from build123d import *

# Parameters (mm, degrees)
SKETCH1_R           = 1.5
SKETCH1_W           = 30
SKETCH1_H           = 8
BOSS_EXTRUDE1_DEPTH = 1.6
SKETCH1_3_W         = 30
SKETCH1_3_H         = 8
BOSS_EXTRUDE2_DEPTH = 11.9


with BuildPart() as part:
    # Sketch1 → Boss-Extrude1 (new body)
    # profile 1 of 2: a face of its own
    with BuildSketch(Plane(origin=(0, 0, 0), x_dir=(0, 1, 0), z_dir=(0, 0, 1))):
        with BuildLine():
            ThreePointArc((0, 2.5), (0.732233047, 0.732233047), (2.5, 0))
            Line((2.5, 0), (5.875, 0))
            Line((5.875, 0), (5.875, 8))
            Line((5.875, 8), (35.875, 8))
            Line((35.875, 8), (35.875, 0))
            Line((35.875, 0), (39.25, 0))
            ThreePointArc((39.25, 0), (41.017766953, 0.732233047), (41.75, 2.5))
            Line((41.75, 2.5), (41.75, 45.6))
            ThreePointArc((41.75, 45.6), (41.017766953, 47.367766953), (39.25, 48.1))
            Line((39.25, 48.1), (2.5, 48.1))
            ThreePointArc((2.5, 48.1), (0.732233047, 47.367766953), (0, 45.6))
            Line((0, 45.6), (0, 2.5))
        make_face()
        with Locations(Location((2.549913685, 2.549913685, 0), (0, 0, 270))):
            Circle(SKETCH1_R, mode=Mode.SUBTRACT)
        with Locations(Location((39.200086315, 2.549913685, 0), (0, 0, 270))):
            Circle(SKETCH1_R, mode=Mode.SUBTRACT)
        with Locations(Location((2.549913685, 45.550086315, 0), (0, 0, 270))):
            Circle(SKETCH1_R, mode=Mode.SUBTRACT)
        with Locations(Location((39.200086315, 45.550086315, 0), (0, 0, 270))):
            Circle(SKETCH1_R, mode=Mode.SUBTRACT)
    # profile 2 of 2: a face of its own
    with BuildSketch(Plane(origin=(0, 0, 0), x_dir=(0, 1, 0), z_dir=(0, 0, 1))):
        with Locations((20.875, 4)):
            Rectangle(SKETCH1_W, SKETCH1_H)
    extrude(amount=BOSS_EXTRUDE1_DEPTH)

    # Sketch1_3 → Boss-Extrude2 (add)
    with BuildSketch(Plane(origin=(0, 0, 0), x_dir=(0, 1, 0), z_dir=(0, 0, 1))):
        with Locations((20.875, 4)):
            Rectangle(SKETCH1_3_W, SKETCH1_3_H)
    extrude(amount=BOSS_EXTRUDE2_DEPTH)


solid = part.part
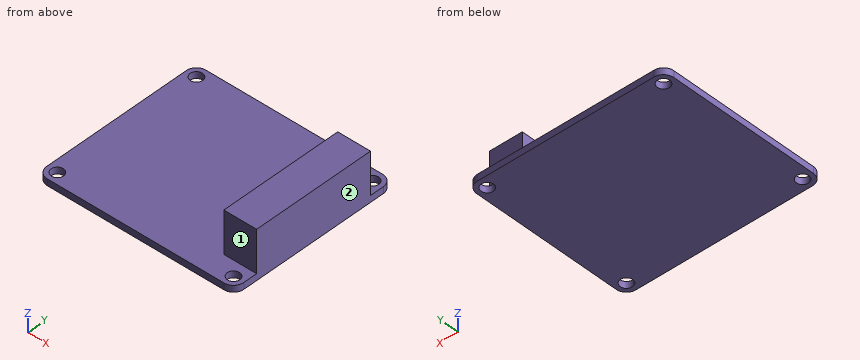
Here's how the part is built. I have some questions about the finished solid (model axes, mm). Face numbers are marked on the shaded views. A direction names the side the tool comes from. Round coordinates to 2 decimals unless told otherwise and drop trailing zeros. Loops run counter-clockwise (first coordinate to the right, second up) from the corner with the lowest first, then second, coordinate; pieces in that order, holes last.
1. Which directions (+Z, -Z, +X, -X, +Y, -Y) give clear straight access to the entire face, cutting with the end or side of a thin tool? Please do the marked faces 1 and 2.
Answer list:
face 1: +Z, +X, -X, -Y
face 2: +Z, -Z, +X, +Y, -Y
2. If we section it at C-C on y = 16: Write out the boundary of the cut face in (x, z).
Answer list:
outline: (-48.1, 0) - (0, 0) - (0, 11.9) - (-8, 11.9) - (-8, 1.6) - (-48.1, 1.6) - close
3. If I drill on line 1 along Z through (x, y) = (-28, 23); line 2 along X through (y, z) = (14.5, 10); line 3 along Y through (x, z) = (-3, 3.5) (3 decimals), over which ranges is the centre line in solid material (lowest first)?
Answer list:
line 1: z = 0 to 1.6
line 2: x = -8 to 0
line 3: y = 5.875 to 35.875
4. If we section it at A-A on x = -6: Write out the boundary of the cut face in (y, z) (3 decimals).
Answer list:
outline: (0, 0) - (41.75, 0) - (41.75, 1.6) - (35.875, 1.6) - (35.875, 11.9) - (5.875, 11.9) - (5.875, 1.6) - (0, 1.6) - close
5. If we section it at B-B on y = 3.5: Write out the boundary of the cut face in (x, z), plus the area to 3 significant figures.
Answer list:
outline: (-48.1, 0) - (-46.71, 0) - (-46.71, 1.6) - (-48.1, 1.6) - close; (-44.39, 0) - (-3.71, 0) - (-3.71, 1.6) - (-44.39, 1.6) - close; (-1.39, 0) - (0, 0) - (0, 1.6) - (-1.39, 1.6) - close
area: 69.5 mm2
6. For P1, Ø4, axis at x = -5.5, z = 6.5, coming from the +Y side (3 decimals); P2, Ø12.5, axis at x = -29, y = 19, coming from the +Z side; P3, Ø2.5, axis at x = -45.55, y = 39.2, coming from the +Z side; P4, Ø6.5, axis at x = -4.5, z = 6, coming from the -Y side (3 decimals), each with a flat end and sliding along its axis, tell me the tip position at first contact or that it passes through.
Answer list:
P1: stops at y = 35.875
P2: stops at z = 1.6
P3: passes through
P4: stops at y = 5.875
7. If we section it at D-D on z = 8.5: Write out the boundary of the cut face in (x, y) (3 decimals), plus the area to 3 significant figures.
Answer list:
outline: (-8, 5.875) - (0, 5.875) - (0, 35.875) - (-8, 35.875) - close
area: 240 mm2
